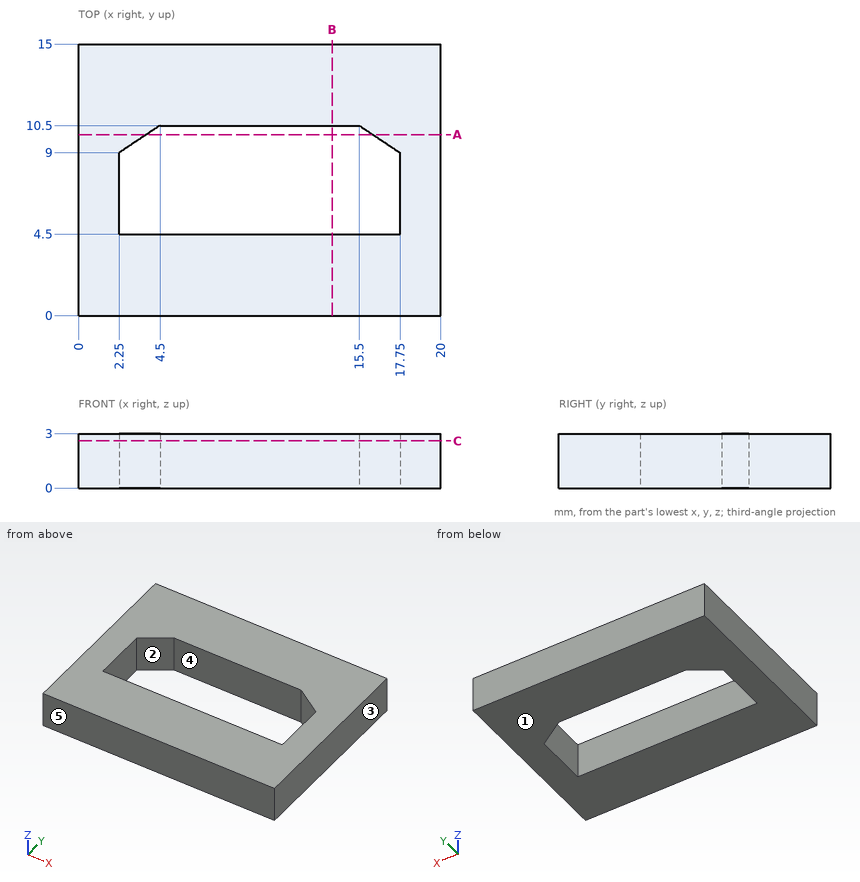
Here's the drawing with two shaded views (mm, measured from the low corner). I have some questions. A direction names the side the tool comes from. Give positions to 0.01 mm unless a question says otherwise; leave off trailing zeros. Loops run counter-clockwise (first coordinate to the right, second up) from the corner with the lowest first, then second, coordinate; pieces in that order, holes last. Notation, with made-up numbers: M 12,-14 L 37,-14 A14 cw 37,8 Z; hole C 43,63 d6. An arc over 180 degrees is marked long. Use one line per item in the form item = value. Start each with the question number.
Q1. Will this pin go through, and if not, where does the flat tip stop? pin 1 Ø1 at (y, z) = (8.5, 1) entering from -X.
Q2. Thinking about a two-plate mould opening in X: for the marked faces 1, 2 and 3, which applies, +X half, -X half, draft (parallel to the pull), parting line (faces both ways), or undercut?
Q3. If we section it at C-C (z = 2.6): Write out the boundary of the cut face in (x, y).
Q4. If we section it at A-A (y = 10): Write out the boundary of the cut face in (x, z), then the cut area to 3 significant figures.
Q5. I need wall thicknesses on line 1 along Y through (x, z) = (8.5, 2.75); line 2 along X through (y, z) = (6.5, 0.6); line 3 along Y through (x, z) = (16.25, 2.3). Which ranges of each line are inside material? Lowest first, please.
Q6. If we section it at B-B (x = 14): Write out the boundary of the cut face in (y, z), then the cut area to 3 significant figures.
Q7. Which directions (+Z, -Z, +X, -X, +Y, -Y) give clear straight access to the entire face, cutting with the end or side of a thin tool? Please do the marked faces 4 and 5.
Taken from the geometry:
q1.pin_1 = 0
q2.face_1 = draft
q2.face_2 = undercut
q2.face_3 = +X half
q3.outline = M 0,0 L 20,0 L 20,15 L 0,15 Z; hole M 2.25,4.5 L 17.75,4.5 L 17.75,9 L 15.5,10.5 L 4.5,10.5 L 2.25,9 Z
q4.outline = M 0,0 L 3.75,0 L 3.75,3 L 0,3 Z; M 16.25,0 L 20,0 L 20,3 L 16.25,3 Z
q4.area = 22.5 mm^2
q5.line_1 = 0 to 4.5, 10.5 to 15
q5.line_2 = 0 to 2.25, 17.75 to 20
q5.line_3 = 0 to 4.5, 10 to 15
q6.outline = M 0,0 L 4.5,0 L 4.5,3 L 0,3 Z; M 10.5,0 L 15,0 L 15,3 L 10.5,3 Z
q6.area = 27.0 mm^2
q7.face_4 = +Z, -Z
q7.face_5 = +Z, -Z, +X, -X, -Y
